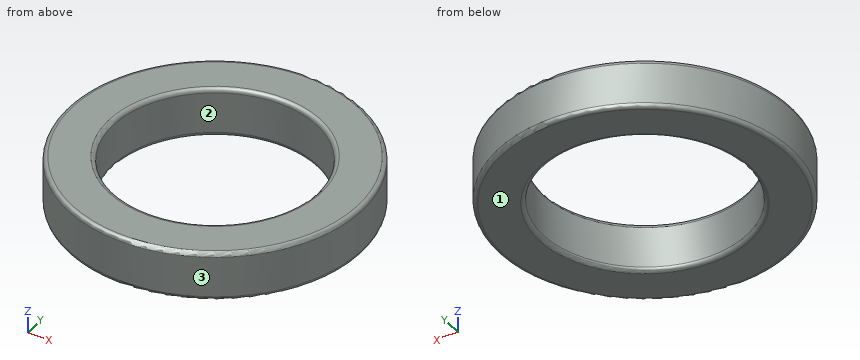
Autodesk Fusion 360 part; units mm, degrees
cylinder "CylinderPrimitive1" add diameter 72 height 12 placed x (1, 0, 0) y (0, 1, 0) z (0, 0, 1) at (0, 0, 0)
hole "Hole1" at (0, 0, 12) direction (0, 0, -1) diameter 50 depth 12 tip angle 180
fillet "Fillet1" radius 1 4 edges at (-33.5638, -13.0182, 12) (-23.3082, 9.0404, 12) (-33.5638, 13.0182, 0) (-23.3082, -9.0404, 0)
Could you check a few things on this model? Use its own coordinates, in mm. Face numbers are marked on the shaded views. Give positions to 0.01 mm unless a question says otherwise; leave off trailing zeros. Order: outer loops, then holes, each group sorted by start corner. A loop starts at its lowest first (then second) coordinate and runs counter-clockwise, first axis right, second up. Notation, with made-up numbers: (-30.75, 41) -> (26.25, 41) arc R26 cw to (26.25, 64) -> close; hole circle Ø11 at (1.5, 37). An arc over 180 degrees is marked (long way). Return JSON: item names as keys, results as strings.
1. Thinking about a two-plate mould opening in Y: for the marked faces 1, 2 and 3, which applies, pulls with the +Y half, pulls with the -Y half, needs draft (parallel to the pull), parting line crosses it, or undercut?
Answer list:
{"face 1": "needs draft", "face 2": "undercut", "face 3": "parting line crosses it"}
2. I need wall thicknesses on line 1 (Y direction, x = 0, z = 8); line 2 (Z direction, x = -12, y = -23); line 3 (Y direction, x = 7, z = 10). Which ranges of each line are inside material? Lowest first, please. Write a range as from..to.
Answer list:
{"line 1": "y = -36..-25, 25..36", "line 2": "z = 0..12", "line 3": "y = -35.31..-24, 24..35.31"}
3. For pin 1 Ø1 at (x, y) = (-18, 16.5) entering from -Z; pin 2 Ø3 at (x, z) = (14.5, 8) entering from +Y; pin 3 Ø1 at (y, z) = (17.5, 1.5) entering from +X, each with a flat end and sliding along its axis, tell me the tip position at first contact or that it passes through.
Answer list:
{"pin 1": "passes through", "pin 2": "stops at y = 33.57", "pin 3": "stops at x = 31.73"}
4. Imagine slicing it at A-A on y = 0. List the corners of the cut face in (x, z) for me.
Answer list:
{"outline": "(-36, 1) arc R1 ccw to (-35, 0) -> (-26, 0) arc R1 ccw to (-25, 1) -> (-25, 11) arc R1 ccw to (-26, 12) -> (-35, 12) arc R1 ccw to (-36, 11) -> close; (25, 1) arc R1 ccw to (26, 0) -> (35, 0) arc R1 ccw to (36, 1) -> (36, 11) arc R1 ccw to (35, 12) -> (26, 12) arc R1 ccw to (25, 11) -> close"}
5. Imagine slicing it at C-C on z = 2.5. List the corners of the cut face in (x, y) for me, then the cut area to 3 significant figures.
Answer list:
{"outline": "circle Ø72 at (0, 0); hole circle Ø50 at (0, 0)", "area": "2,110 mm2"}
